For this review, use the dimensioned drawing (mm, ordinates from the lowest corner) and the shaded views. A direction names the side the tool comes from. Coordinates: 2 decimals unless noted, no trailing zeros.
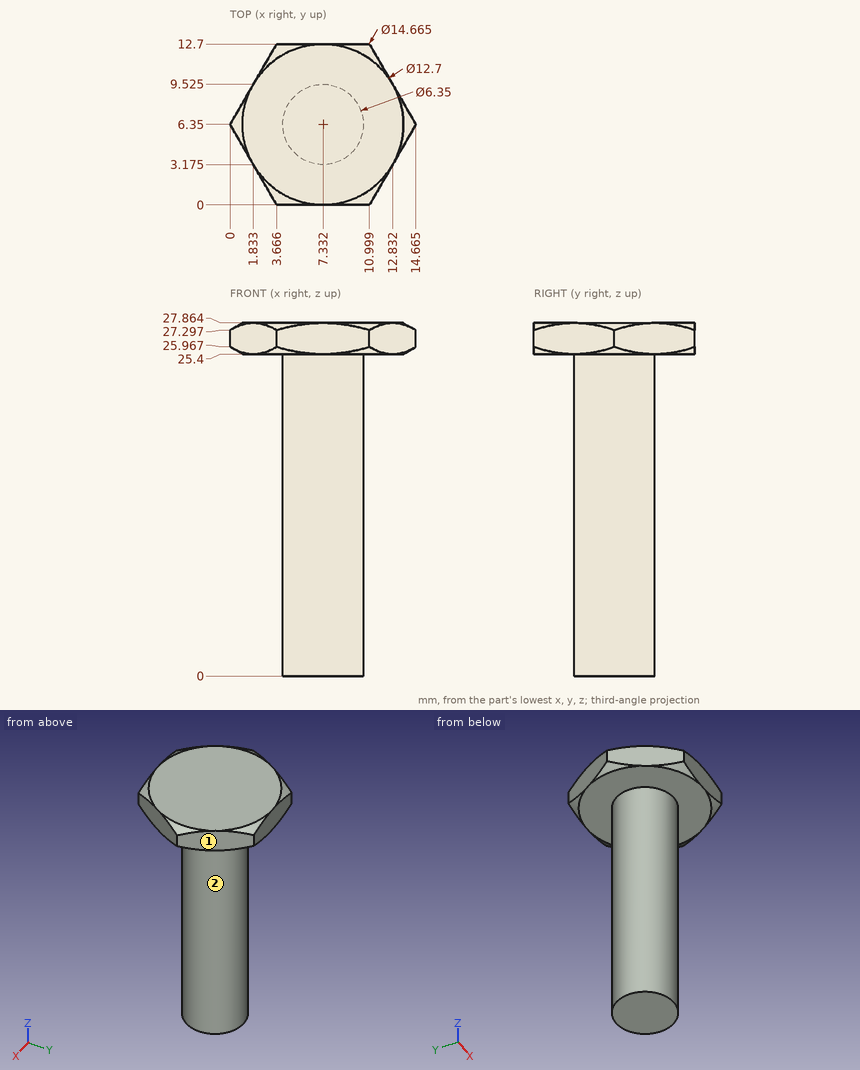
Item 1: Machinability: for the marked faces 1 and 2, which of the approach directions +Z, -Z, +X, -X, +Y, -Y give a long, thin tool a straight path to every point of the face, cutting with its end or side? Answer none if there is none.
Solved:
face 1: +Z, -Z, +X, +Y
face 2: -Z
Item 2: For pin 1 (6 mm diameter, centred on x = 11, z = 8, fed in from -Y); pin 2 (5 mm diameter, centred on y = 7.5, z = 11, fed in from +X), all flat-tipped, find the tip position at first contact; note any pin that passes through.
Solved:
pin 1: stops at y = 3.25
pin 2: stops at x = 10.51
Item 3: To check wall thickness, follow line 1 along Z through (x, y) = (9.25, 11.25); line 2 along X through (y, z) = (6.5, 19.75); line 3 along Y through (x, z) = (5.5, 13.75) (1 decimal). State the ranges of each line that lie inside material, in increasing order.
Solved:
line 1: z = 25.4 to 27.86
line 2: x = 4.16 to 10.5
line 3: y = 3.8 to 8.9
